Study the drawing (mm; zero at the part's minimum x, y, z) and answer. Coordinates: 2 decimals unless noted, no trailing zeros. Order: outer loops, then holes, each group sorted by start corner. A loop starts at its lowest first (then second) coordinate and runs counter-clockwise, first axis right, second up. Notation, with made-up numbers: (43, 77) -> (66, 77) arc R32 ccw to (66, 103) -> close; hole circle Ø3 at (63.5, 85.5). An arc over 180 degrees is marked (long way). One line per question, with ' | ' between items.
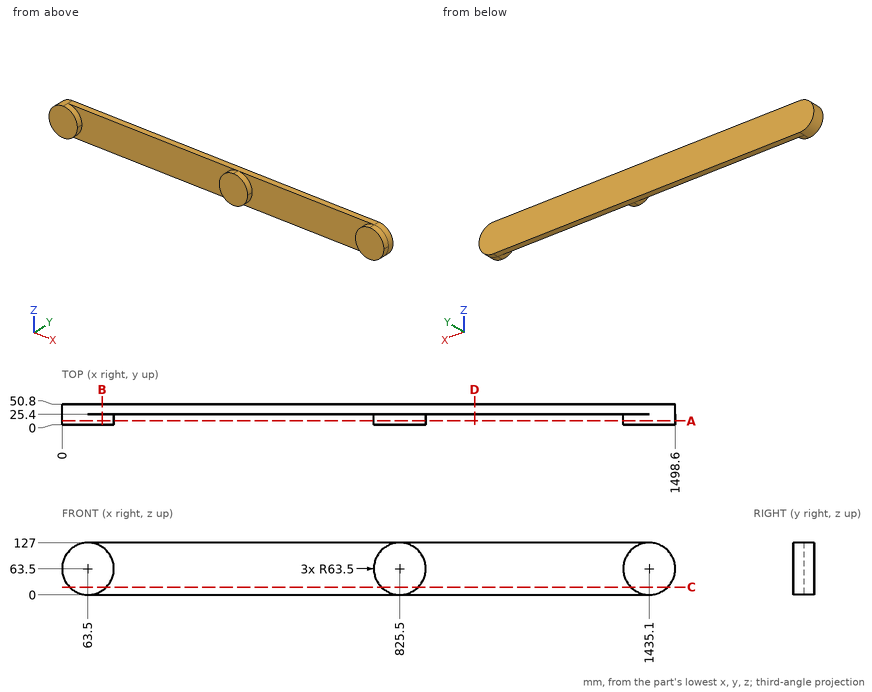
Item 1: Section C-C, the plane z = 18.5 is taken. Give the vertices of the cut face in (x, y).
Computed values:
outline: (18.7, 0) -> (108.3, 0) -> (108.3, 25.4) -> (780.7, 25.4) -> (780.7, 0) -> (870.3, 0) -> (870.3, 25.4) -> (1390.3, 25.4) -> (1390.3, 0) -> (1479.9, 0) -> (1479.9, 50.8) -> (18.7, 50.8) -> close
Item 2: Section A-A, the plane y = 9.5 is taken. Give the vertices of the cut face in (x, z), plus the area to 3 significant figures.
Computed values:
outline: (63.5, 0) arc R63.5 ccw to (127, 63.5) arc R63.5 ccw to (63.5, 127) arc R63.5 ccw to start; (825.5, 0) arc R63.5 ccw to (889, 63.5) arc R63.5 ccw to (825.5, 127) arc R63.5 ccw to start; (1435.1, 0) arc R63.5 ccw to (1498.6, 63.5) arc R63.5 ccw to (1435.1, 127) arc R63.5 ccw to start | area: 38,000 mm^2
Item 3: Find the intervals of material crossed by L1, parallel to X at y = 22, z = 62; L2, parallel to X at y = 23, z = 20.5; L3, parallel to Y at x = 393, z = 84, in increasing order.
Computed values:
L1: x = 0.02 to 126.98, 762.02 to 888.98, 1371.62 to 1498.58 | L2: x = 16.77 to 110.23, 778.77 to 872.23, 1388.37 to 1481.83 | L3: y = 25.4 to 50.8
Item 4: Section B-B, the plane x = 98 is taken. Give the vertices of the cut face in (y, z), plus the area to 3 significant figures.
Computed values:
outline: (0, 10.19) -> (25.4, 10.19) -> (25.4, 0) -> (50.8, 0) -> (50.8, 127) -> (25.4, 127) -> (25.4, 116.81) -> (0, 116.81) -> close | area: 5,930 mm^2
Item 5: Each of these flat-tipped pins is pushed along its axis until it touches: pin 1 Ø8 at (y, z) = (35.5, 87.5) entering from -X; pin 2 Ø1 at (x, z) = (1098.5, 106) entering from -Y; pin 3 Ø8 at (y, z) = (11.5, 95.5) entering from +X; pin 4 Ø12 at (x, y) = (558, 16.5) entering from +Z. Where does it stop, or does it pass through?
Computed values:
pin 1: stops at x = 3.23 | pin 2: stops at y = 25.4 | pin 3: stops at x = 1492.09 | pin 4: passes through
Item 6: Section D-D, the plane x = 1008.5 is taken. Give the vertices of the cut face in (y, z).
Computed values:
outline: (25.4, 0) -> (50.8, 0) -> (50.8, 127) -> (25.4, 127) -> close
